Design review of the part built by this model. Coordinates are the model's own, in mm. Face numbers are marked on the shaded views. A direction names the side the tool comes from. Round coordinates to 2 decimals unless told otherwise and drop trailing zeros. Loops run counter-clockwise (first coordinate to the right, second up) from the corner with the lowest first, then second, coordinate; pieces in that order, holes last. Notation, with made-up numbers: (43, -16) -> (63, -16) arc R32 cw to (63, 15) -> close; hole circle Ø9 at (-24.75, 55.5). An arc over 180 degrees is marked (long way). Use a Markdown table: item, result. Add a question column.
Autodesk Inventor part; units mm, degrees
ref_plane "YZ Plane" through (0, 0, 0) normal (1, 0, 0) x (0, 1, 0)
ref_plane "XZ Plane" through (0, 0, 0) normal (0, 1, 0) x (-1, 0, 0)
ref_plane "XY Plane" through (0, 0, 0) normal (0, 0, 1) x (1, 0, 0)
sketch "Sketch1" plane through (0, 0, 0) normal (0, 1, 0) x (-1, 0, 0)
  circle A0 centre (0, 0) radius 15.55
  dimension "d1" = 31.1
extrude "Extrusion1" add sketch "Sketch1" along normal blind 18.4
sketch "Sketch2" plane through (0, 18.4, 0) normal (0, 1, 0) x (1, 0, 0)
  circle A0 centre (0, 0) radius 22.7
  dimension "d4" = 45.4
extrude "Extrusion2" add sketch "Sketch2" along normal blind 6.4
sketch "Sketch3" plane through (0, 24.8, 0) normal (0, 1, 0) x (1, 0, 0)
  circle A0 centre (0, 0) radius 24.25
  dimension "d7" = 48.5
extrude "Extrusion3" add sketch "Sketch3" along normal blind 9.4
sketch "Sketch4" plane through (0, 0, 0) normal (0, -1, 0) x (1, 0, 0)
  circle A0 centre (0, 0) radius 22.7
extrude "Extrusion4" add sketch "Sketch4" along normal blind 6.4
sketch "Sketch5" plane through (0, -6.4, 0) normal (0, -1, 0) x (1, 0, 0)
  circle A0 centre (0, 0) radius 24.25
extrude "Extrusion5" add sketch "Sketch5" along normal blind 9.4
chamfer "Chamfer1" distance 3 angle 45 1 edges at (-24.25, 34.2, 0)
chamfer "Chamfer2" distance 3 angle 45 1 edges at (-24.25, -15.8, 0)
properties part number "Hydraulic cylinder part 2"
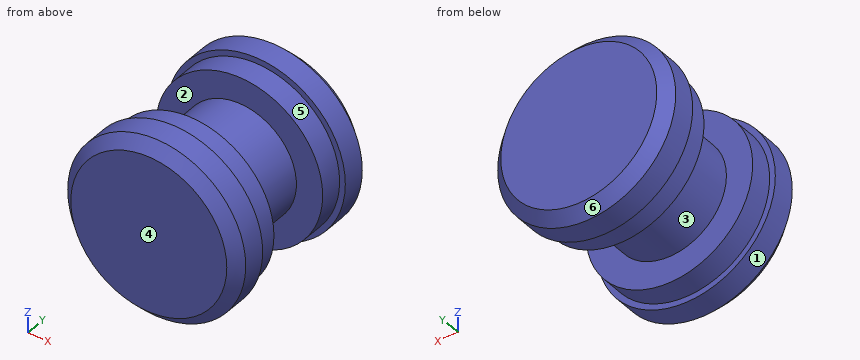
1. For the marked faces 5 and 6, list the 3-axis set-ups (+Z, -Z, +X, -X, +Y, -Y) from which the entire face can be reached by the end or side of a thin tool; tool diameter is ignored.
2. Insertion check: P1, Ø3, axis at y = -9.5, z = 11, coming from the +X side; P2, Ø5, axis at x = -11, y = 4.5, coming from the -Z side; P3, Ø3, axis at y = 28, z = -18, coming from the -X side. Each pin has a flat end and moves straight along its axis. Give the tip position at first contact, or say it passes through.
3. Consider section D-D on y = -1.5. State the section outline as (x, z) points, plus the area to 3 significant figures.
4. Consider section B-B on x = 0. State the section outline as (y, z) points, plus the area to 3 significant figures.
5. Mouldability with a two-part tool opening along Y and no side actions: class the marked faces 1, 2, 3 and 4 as +Y half, -Y half, draft (parallel to the pull), parting line (faces both ways), or undercut.
6. Consider section C-C on y = -12. State the section outline as (x, z) points.
7. Consider section A-A on z = 0. State the section outline as (x, y) points, plus the area to 3 significant figures.
8. To check wall thickness, follow probe 1 along Y at (x, z) = (8.5, -15.5); probe 2 along Z at (x, y) = (0, 18); probe 3 along X at (y, z) = (-6.5, 8.5). State the ranges of each line that lie inside material, in increasing order. Write a range as from..to.
Verdict:
| question | item | result |
|---|---|---|
| 1 | face 5 | none |
| 1 | face 6 | +Y |
| 2 | P1 | stops at x = 22.31 |
| 2 | P2 | stops at z = -13.02 |
| 2 | P3 | stops at x = -17.77 |
| 3 | outline | circle Ø45.4 at (0, 0) |
| 3 | area | 1,620 mm² |
| 4 | outline | (-15.8, -21.25) -> (-12.8, -24.25) -> (-6.4, -24.25) -> (-6.4, -22.7) -> (0, -22.7) -> (0, -15.55) -> (18.4, -15.55) -> (18.4, -22.7) -> (24.8, -22.7) -> (24.8, -24.25) -> (31.2, -24.25) -> (34.2, -21.25) -> (34.2, 21.25) -> (31.2, 24.25) -> (24.8, 24.25) -> (24.8, 22.7) -> (18.4, 22.7) -> (18.4, 15.55) -> (0, 15.55) -> (0, 22.7) -> (-6.4, 22.7) -> (-6.4, 24.25) -> (-12.8, 24.25) -> (-15.8, 21.25) -> close |
| 4 | area | 2,050 mm² |
| 5 | face 1 | draft |
| 5 | face 2 | undercut |
| 5 | face 3 | undercut |
| 5 | face 4 | -Y half |
| 6 | outline | circle Ø48.5 at (0, 0) |
| 7 | outline | (-24.25, -12.8) -> (-21.25, -15.8) -> (21.25, -15.8) -> (24.25, -12.8) -> (24.25, -6.4) -> (22.7, -6.4) -> (22.7, 0) -> (15.55, 0) -> (15.55, 18.4) -> (22.7, 18.4) -> (22.7, 24.8) -> (24.25, 24.8) -> (24.25, 31.2) -> (21.25, 34.2) -> (-21.25, 34.2) -> (-24.25, 31.2) -> (-24.25, 24.8) -> (-22.7, 24.8) -> (-22.7, 18.4) -> (-15.55, 18.4) -> (-15.55, 0) -> (-22.7, 0) -> (-22.7, -6.4) -> (-24.25, -6.4) -> close |
| 7 | area | 2,050 mm² |
| 8 | probe 1 | y = -15.8..0, 18.4..34.2 |
| 8 | probe 2 | z = -15.55..15.55 |
| 8 | probe 3 | x = -22.71..22.71 |
